Could you check a few things on this model? Use its own coordinates, in mm. A direction names the side the tool comes from. Coordinates: 2 decimals unless noted, no trailing zeros. Loops run counter-clockwise (first coordinate to the right, second up) from the corner with the lowest first, then second, coordinate; pieces in that order, holes last. Notation, with made-up numbers: (-15, -25) -> (28, -25) arc R31 ccw to (28, 6) -> close; hole circle Ø7 at (57, 2.5). An arc over 180 degrees is marked (long way). One line per question, with ' | ' between items.
```python
from build123d import *

# Parameters (mm, degrees)
F0_R     = 15
F4_DEPTH = 25
F1_R     = 30
F5_DEPTH = 25
F2_SIZE  = 10
F3_SIZE  = 5


with BuildPart() as f4:
    # F0 (on Right) → F4 (new body)
    with BuildSketch(Plane.YZ):
        Circle(F0_R)
    extrude(amount=F4_DEPTH)

    # F1 (on face) → F5 (join)
    with BuildSketch(Plane.YZ.offset(25)):
        Circle(F1_R)
    extrude(amount=F5_DEPTH)

    # F2
    f2_edges = [f4.edges().sort_by_distance(p)[0] for p in [
        (50, -30, 0),
    ]]
    chamfer(f2_edges, length=F2_SIZE)

    # F3
    f3_edges = [f4.edges().sort_by_distance(p)[0] for p in [
        (25, -30, 0),
    ]]
    chamfer(f3_edges, length=F3_SIZE)


solid = f4.part
```
Q1. For faces 3 (the face through (50, 0, 0)), 4 (the face through (12.325, -14.985, 0.66)), which set-ups out of +Z, -Z, +X, -X, +Y, -Y let a thin tool reach every point of the face, with its end or its side?
Values follow:
face 3: +Z, -Z, +X, +Y, -Y | face 4: -X
Q2. Imagine slicing it at A-A on y = 0. Write out the boundary of the cut face in (x, z).
Values follow:
outline: (0, -15) -> (25, -15) -> (25, -25) -> (30, -30) -> (40, -30) -> (50, -20) -> (50, 20) -> (40, 30) -> (30, 30) -> (25, 25) -> (25, 15) -> (0, 15) -> close
Q3. Please list where these lines run through material, in increasing order: L1, parallel to X at y = -18, z = 3; L2, parallel to Y at x = 44.5, z = -2; L3, parallel to Y at x = 6.5, z = -2.5. Write a range as [from, to].
Values follow:
L1: x = [25, 50] | L2: y = [-25.42, 25.42] | L3: y = [-14.79, 14.79]
Q4. Imagine slicing it at C-C on x = 42. Write out the boundary of the cut face in (y, z).
Values follow:
outline: circle Ø56 at (0, 0)
Q5. For pin 1 (1.5 mm diameter, centred on y = -15, z = 20.5, fed in from +X); pin 2 (1.5 mm diameter, centred on x = 17.5, z = 13.5, fed in from +Y); pin 3 (12 mm diameter, centred on y = 18.5, z = -22.5, fed in from -X), each with a flat end and sliding along its axis, tell me the tip position at first contact or that it passes through.
Values follow:
pin 1: stops at x = 45.35 | pin 2: stops at y = 7.9 | pin 3: stops at x = 25
Q6. Imagine slicing it at D-D on x = 5. Write out the boundary of the cut face in (y, z).
Values follow:
outline: circle Ø30 at (0, 0)
Q7. We'd pull the mould along Y, two halves only. Please class faces 1 (the face through (25, 11, -11)), 2 (the face through (25.243, 24.077, 7.582)): released by +Y, released by -Y, zero draft, split by the parting line, or undercut.
Values follow:
face 1: zero draft | face 2: split by the parting line
